Input: part model. Units: mm. Frame: model coordinates. Face numbers are marked on the shaded views. A direction names the side the tool comes from. Coordinates: 2 decimals unless noted, no trailing zeros. Order: outer loops, then holes, each group sorted by start corner. A loop starts at its lowest first (then second) coordinate and runs counter-clockwise, first axis right, second up. Notation, with made-up numbers: (-12.5, 67) -> (42.5, 67) arc R22 ccw to (42.5, 84) -> close; hole circle Ø8 at (-11, 34). An arc over 180 degrees is marked (long way). Write each question's results on one line, items separated by ' | '.
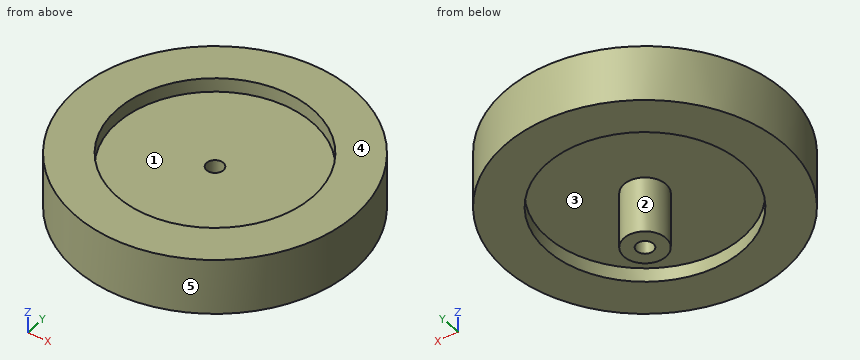
```python
from build123d import *

# Parameters (mm, degrees)
SKETCH1_R           = 50
BOSS_EXTRUDE1_DEPTH = 10
SKETCH2_R           = 35
CUT_EXTRUDE1_DEPTH  = 5
SKETCH3_R           = 7.5
BOSS_EXTRUDE2_DEPTH = 20
CUT_EXTRUDE2_REACH  = 37
SKETCH4_R           = 3


with BuildPart() as part:
    # Sketch1 → Boss-Extrude1 (new body, symmetric)
    with BuildSketch(Plane.XY):
        Circle(SKETCH1_R)
    extrude(amount=BOSS_EXTRUDE1_DEPTH, both=True)

    # Sketch2 → Cut-Extrude1 (cut)
    with BuildSketch(Plane.XY.offset(10)):
        Circle(SKETCH2_R)
    cut_extrude1 = extrude(amount=-CUT_EXTRUDE1_DEPTH, mode=Mode.SUBTRACT)

    # Mirror1: Cut-Extrude1 across plane
    add(cut_extrude1.mirror(Plane.XY), mode=Mode.SUBTRACT)

    # Sketch3 → Boss-Extrude2 (add)
    with BuildSketch(Plane(origin=(0, 0, -5), x_dir=(-1, 0, 0), z_dir=(0, 0, -1))):
        Circle(SKETCH3_R)
    extrude(amount=BOSS_EXTRUDE2_DEPTH)

    # Sketch4 → Cut-Extrude2 (cut, up to next)
    with BuildSketch(Plane(origin=(0, 0, -25), x_dir=(-1, 0, 0), z_dir=(0, 0, -1)), mode=Mode.PRIVATE) as cut_extrude2_sk1:
        Circle(SKETCH4_R)
    cut_extrude2_tool1 = extrude(cut_extrude2_sk1.sketch, amount=-CUT_EXTRUDE2_REACH, mode=Mode.PRIVATE) & part.part
    add(cut_extrude2_tool1.solids().sort_by_distance((0, 0, -25))[0], mode=Mode.SUBTRACT)


solid = part.part
```
(1) Mould query, pull axis Y, two halves, no side actions, for the marked faces 3, 4 and 5. Classes: +Y half, -Y half, draft (parallel to the pull), parting line (faces both ways), or undercut.
Return value:
face 3: undercut | face 4: draft | face 5: parting line
(2) Line query: line 1 along Y through (x, z) = (0, -8.7); line 2 along Y through (x, z) = (0, 7.75); line 3 along Z through (x, y) = (25.5, -10.5). Output: solid intervals per line, ascending. Write a range as from..to.
Return value:
line 1: -50..-35, -7.5..-3, 3..7.5, 35..50 | line 2: -50..-35, 35..50 | line 3: -5..5
(3) Pin query (flat end, axial travel): P1, Ø12, axis at y = 8.5, z = -5.5, coming from the +X side; P2, Ø5, axis at x = 20.5, z = -10.5, coming from the +Y side; P3, Ø5, axis at x = 26, z = -4.5, coming from the -Y side. Return the tip coordinate at first contact, or that it passes through.
Return value:
P1: x = 49.94 | P2: y = 46.63 | P3: y = -44.13
(4) Cut plane D-D, the plane x = 25. Return loops of the section in (y, z), plus the area to 3 significant figures.
Return value:
outline: (-43.3, -10) -> (-24.49, -10) -> (-24.49, -5) -> (24.49, -5) -> (24.49, -10) -> (43.3, -10) -> (43.3, 10) -> (24.49, 10) -> (24.49, 5) -> (-24.49, 5) -> (-24.49, 10) -> (-43.3, 10) -> close | area: 1,240 mm2
(5) Cut plane C-C, the plane z = 0. Return loops of the section in (x, y).
Return value:
outline: circle Ø100 at (0, 0); hole circle Ø6 at (0, 0)
(6) Reachability of the marked faces 1 and 2 from +Z, -Z, +X, -X, +Y, -Y: full face, straight path, thin tool, end or side. Return the list, or none.
Return value:
face 1: +Z | face 2: -Z
(7) Cut plane A-A, the plane y = 0. Return loops of the section in (x, z).
Return value:
outline: (-50, -10) -> (-35, -10) -> (-35, -5) -> (-7.5, -5) -> (-7.5, -25) -> (-3, -25) -> (-3, 5) -> (-35, 5) -> (-35, 10) -> (-50, 10) -> close; (3, -25) -> (7.5, -25) -> (7.5, -5) -> (35, -5) -> (35, -10) -> (50, -10) -> (50, 10) -> (35, 10) -> (35, 5) -> (3, 5) -> close
